from build123d import *

# Parameters (mm, degrees)
BOSS_EXTRUDE1_DEPTH   = 10
BOSS_EXTRUDE1_2_DEPTH = 10
BOSS_EXTRUDE1_3_DEPTH = 10
SKETCH3_W             = 13
SKETCH3_H             = 24
BOSS_EXTRUDE2_DEPTH   = 5
SKETCH4_W             = 6
SKETCH4_H             = 13
BOSS_EXTRUDE3_DEPTH   = 42
SKETCH5_W             = 6
SKETCH5_H             = 24
BOSS_EXTRUDE4_DEPTH   = 2
SKETCH6_R             = 1.6
CUT_EXTRUDE1_DEPTH    = 60.575582246
SKETCH8_W             = 15
SKETCH8_H             = 24
BOSS_EXTRUDE5_DEPTH   = 3
SKETCH7_W             = 5.75
SKETCH7_H             = 2.65
CUT_EXTRUDE2_DEPTH    = 12.5


with BuildPart() as part:
    # Sketch2 → Boss-Extrude1 (new body)
    with BuildSketch(Plane.XY):
        with BuildLine():
            Line((-26.5, 0), (-30.65, 0))
            Line((-30.65, 0), (-32.618157491, 0))
            Line((-32.618157491, 0), (-31.015837104, 1.142896884))
            ThreePointArc((-31.015837104, 1.142896884), (-29.165912572, 3.280355677), (-28.5, 6.027629109))
            Line((-28.5, 6.027629109), (-28.5, 24))
            Line((-28.5, 24), (-26.5, 24))
            Line((-26.5, 24), (-26.5, 0))
        make_face()
    extrude(amount=BOSS_EXTRUDE1_DEPTH)



with BuildPart() as body_2:
    # Sketch2 → Boss-Extrude1 2 (new body)
    with BuildSketch(Plane.XY):
        with BuildLine():
            Line((-31, 24), (-39.5, 24))
            Line((-39.5, 24), (-39.5, 8.68))
            Line((-39.5, 8.68), (-39.5, 6.362551494))
            Line((-39.5, 6.362551494), (-38.492686138, 8.449627525))
            ThreePointArc((-38.492686138, 8.449627525), (-37.750547948, 9.507229314), (-36.71, 10.273095232))
            Line((-36.71, 10.273095232), (-31, 13.19))
            Line((-31, 13.19), (-31, 24))
        make_face()
    extrude(amount=BOSS_EXTRUDE1_2_DEPTH)


with BuildPart() as body_3:
    # Sketch2 → Boss-Extrude1 3 (new body)
    with BuildSketch(Plane.XY):
        with BuildLine():
            Line((-30.2, 5.530404879), (-30.2, 11.689701848))
            Line((-30.2, 11.689701848), (-35.685050881, 8.887710417))
            ThreePointArc((-35.685050881, 8.887710417), (-35.938141024, 2.314923436), (-30.2, 5.530404879))
        make_face()
    extrude(amount=BOSS_EXTRUDE1_3_DEPTH)


with BuildPart() as part_1:
    add(part.part)

    add(body_2.part)  # Boss-Extrude2 merges body 2

    add(body_3.part)  # Boss-Extrude2 merges body 3
    # Sketch3 → Boss-Extrude2 (add)
    with BuildSketch(Plane.XY.offset(10)):
        with Locations((-33, 12)):
            Rectangle(SKETCH3_W, SKETCH3_H)
    extrude(amount=BOSS_EXTRUDE2_DEPTH)

    # Sketch4 → Boss-Extrude3 (add)
    with BuildSketch(Plane(origin=(0, 24, 0), x_dir=(1, 0, 0), z_dir=(0, 1, 0))):
        with Locations((-23.5, -8.5)):
            Rectangle(SKETCH4_W, SKETCH4_H)
    extrude(amount=-BOSS_EXTRUDE3_DEPTH)

    # Sketch5 → Boss-Extrude4 (add)
    with BuildSketch(Plane(origin=(0, 0, 2), x_dir=(-1, 0, 0), z_dir=(0, 0, -1))):
        with Locations((23.5, 12)):
            Rectangle(SKETCH5_W, SKETCH5_H)
    extrude(amount=BOSS_EXTRUDE4_DEPTH)

    # Sketch6 → Cut-Extrude1 (cut, through all)
    with BuildSketch(Plane.XZ.offset(18)):
        with Locations(Location((-23.5, 8.5, 0), (0, 0, 270))):
            Circle(SKETCH6_R)
    extrude(amount=-CUT_EXTRUDE1_DEPTH, mode=Mode.SUBTRACT)

    # Sketch8 → Boss-Extrude5 (add)
    with BuildSketch(Plane(origin=(-20.5, 0, 0), x_dir=(0, 0, -1), z_dir=(1, 0, 0))):
        with Locations((-7.5, 12)):
            Rectangle(SKETCH8_W, SKETCH8_H)
    extrude(amount=BOSS_EXTRUDE5_DEPTH)

    # Sketch7 → Cut-Extrude2 (cut)
    with BuildSketch(Plane(origin=(0, 0, 0), x_dir=(-1, 0, 0), z_dir=(0, 0, -1))):
        with Locations((23.5, 3.325)):
            Rectangle(SKETCH7_W, SKETCH7_H)
    extrude(amount=-CUT_EXTRUDE2_DEPTH, mode=Mode.SUBTRACT)


solid = part_1.part
Work out the finished part from the listing and answer in its coordinate system (mm). A direction names the side the tool comes from. Round coordinates to 2 decimals unless told otherwise and drop trailing zeros. Loops run counter-clockwise (first coordinate to the right, second up) from the corner with the lowest first, then second, coordinate; pieces in that order, holes last. Notation, with made-up numbers: (0, -21) - (58, -21) arc R20 cw to (58, 5) - close; hole circle Ø6 at (-17, 33). An arc over 180 degrees is marked (long way). Use one line per item in the form item = value. Start each with the question number.
(1) Find section B-B on x = -23.5. Determine the outline of the cut face in (y, z), and give its area (3 significant figures).
(2) Determine the mould class of faces 4 (the face through (-31, 19, 5)), 5 (the face through (-21.914, 14.19, 8.708)), 6 (the face through (-29, 7, 15)) for opening direction Z: +Z half, -Z half, draft (parallel to the pull), parting line (faces both ways), or undercut.
(3) Which of the six approach directions +Z, -Z, +X, -X, +Y, -Y give full straight-line access (tool end or side, diameter ignored) to faces 1 (the face through (-24, -9, 2)), 2 (the face through (-33.895, 11.711, 4.93)), 3 (the face through (-31.83, 0.56, 4.93))?
(4) Find section D-D on z = 4. Determine the outline of the cut face in (x, y) (3 decimals).
(5) Find section A-A on z = 8.5. Give the number of separate pieces and of enclosed holes in the cut face, and give its area (3 significant figures).
(6) Consider line 1 (X direction, y = 14.5, z = 8.5); line 2 (X direction, y = -7.5, z = 8.5); line 3 (X direction, y = 11.25, z = 8.5). Determine where each line is inside the solid, lowest interval first.
(7) Flat-ended cylindrical pins translate along their axes: P1, Ø2, axis at x = -34, y = 13, coming from the -Z side; P2, Ø4, axis at x = -32, z = 7, coming from the -Y side; P3, Ø2, axis at y = 3.5, z = 7.5, coming from the -X side; P4, Ø4, axis at y = -11, z = 6.5, coming from the +X side. Find the tip coordinate at first contact, or state that the pin passes through.
(8) Find section C-C on y = 19.5. Determine the outline of the cut face in (x, z), and give its area (3 significant figures).
Answer list:
q1.outline = (-18, 2) - (0, 2) - (0, 0) - (2, 0) - (2, 6.9) - (-18, 6.9) - close; (-18, 10.1) - (2, 10.1) - (2, 12.5) - (4.65, 12.5) - (4.65, 10.1) - (24, 10.1) - (24, 15) - (-18, 15) - close; (4.65, 0) - (24, 0) - (24, 6.9) - (4.65, 6.9) - close
q1.area = 435 mm^2
q2.face_4 = draft
q2.face_5 = undercut
q2.face_6 = +Z half
q3.face_1 = -Z, +X, -X, -Y
q3.face_2 = -Z
q3.face_3 = -Z, -X
q4.outline = (-39.5, 6.363) - (-38.493, 8.45) arc R4 cw to (-36.71, 10.273) - (-31, 13.19) - (-31, 24) - (-39.5, 24) - close; (-35.685, 8.888) arc R3.77 ccw (long way) to (-30.2, 5.53) - (-30.2, 11.69) - close; (-32.618, 0) - (-26.5, 0) - (-26.5, -18) - (-20.5, -18) - (-20.5, 0) - (-17.5, 0) - (-17.5, 24) - (-28.5, 24) - (-28.5, 6.028) arc R6 cw to (-31.016, 1.143) - close; hole (-26.375, 2) - (-20.625, 2) - (-20.625, 4.65) - (-26.375, 4.65) - close
q5.separate_pieces = 4
q5.enclosed_holes = 0
q5.area = 404 mm^2
q6.line_1 = -39.5 to -31, -28.5 to -25.1, -21.9 to -17.5
q6.line_2 = -26.5 to -25.1, -21.9 to -20.5
q6.line_3 = -39.5 to -34.8, -31.06 to -30.2, -28.5 to -25.1, -21.9 to -17.5
q7.P1 = 0
q7.P2 = 0
q7.P3 = -37.6
q7.P4 = -20.5
q8.outline = (-39.5, 0) - (-31, 0) - (-31, 10) - (-28.5, 10) - (-28.5, 0) - (-17.5, 0) - (-17.5, 15) - (-39.5, 15) - close; hole circle Ø3.2 at (-23.5, 8.5)
q8.area = 297 mm^2
